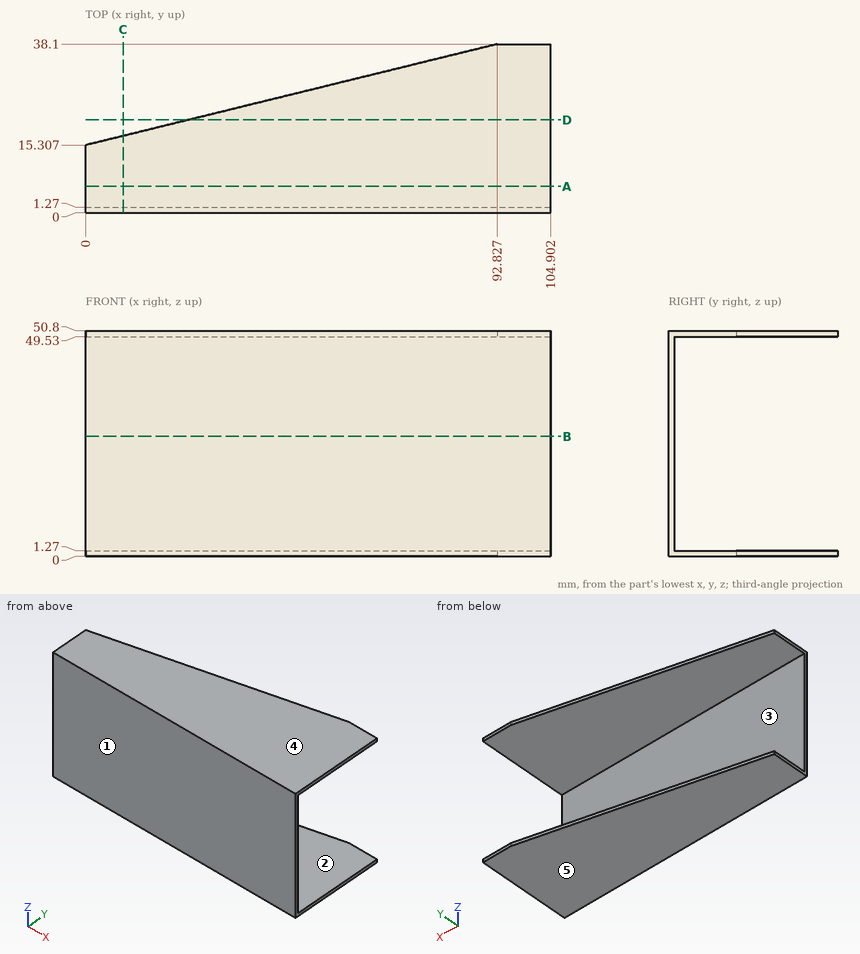
Part print with two shaded views. Sizes in mm from the minimum x, y, z corner. A direction names the side the tool comes from. Give positions to 0.01 mm unless a question says otherwise; leave off trailing zeros. Order: outer loops, then holes, each group sorted by start corner. A loop starts at its lowest first (then second) coordinate and runs counter-clockwise, first axis right, second up. Notation, with made-up numbers: M -36.75,-35.75 L -28.75,-35.75 A22 ccw -28.75,-24.75 Z; hole C 67.5,-39 d9. An arc over 180 degrees is marked long. Put each result on its own line as item: value.
Item 1: Cut at A-A on y = 6. Write the cut outline in (x, z).
Results are:
outline: M 0,0 L 104.9,0 L 104.9,1.27 L 0,1.27 Z; M 0,49.53 L 104.9,49.53 L 104.9,50.8 L 0,50.8 Z
Item 2: Pull direction Z, two halves, no side cores. Call the marked faces 3, 4 and 5: +Z half, -Z half, draft (parallel to the pull), parting line (faces both ways), or undercut.
Results are:
face 3: undercut
face 4: +Z half
face 5: -Z half
Item 3: Wall check: probe 1 along Z at (x, y) = (88.5, 9.5); probe 2 along Y at (x, z) = (84.5, 4). Give the ranges that are in metal, low to high.
Results are:
probe 1: 0 to 1.27, 49.53 to 50.8
probe 2: 0 to 1.27
Item 4: Cut at C-C on x = 8.5. Write the cut outline in (y, z).
Results are:
outline: M 0,0 L 17.39,0 L 17.39,1.27 L 1.27,1.27 L 1.27,49.53 L 17.39,49.53 L 17.39,50.8 L 0,50.8 Z
Item 5: Drop a flat-ended pin along its axis: pin 1 Ø4 at (x, z) = (58.5, 8) entering from +Y. Give the stop position or say it passes through.
Results are:
pin 1: y = 1.27
Item 6: Cut at D-D on y = 21. Write the cut outline in (x, z) (1 decimal).
Results are:
outline: M 23.2,0 L 104.9,0 L 104.9,1.3 L 23.2,1.3 Z; M 23.2,49.5 L 104.9,49.5 L 104.9,50.8 L 23.2,50.8 Z
Item 7: Which spindle directions (+Z, -Z, +X, -X, +Y, -Y) get a long thin tool onto all of the face, cutting with end or side? Do the marked faces 1 and 2. Say none if no direction does.
Results are:
face 1: +Z, -Z, +X, -X, -Y
face 2: +X, -X, +Y
Item 8: Cut at B-B on z = 27. Write the cut outline in (x, y), then the cut area to 3 significant figures.
Results are:
outline: M 0,0 L 104.9,0 L 104.9,1.27 L 0,1.27 Z
area: 133 mm2
